```python
from build123d import *

# Parameters (mm, degrees)
F0_R     = 32.397128
F1_DEPTH = 25.4


with BuildPart() as f1:
    # F0 (on Top) → F1 (new body)
    with BuildSketch(Plane.XY):
        with Locations((37.62687, 37.525859)):
            Circle(F0_R)
        with BuildLine():
            ThreePointArc((64.038143, 27.863669), (55.546064, 15.850626), (42.150506, 9.768879))
            Line((42.150506, 9.768879), (57.342436, 32.889675))
            Line((57.342436, 32.889675), (17.938334, 32.889675))
            Line((17.938334, 32.889675), (33.3534, 9.729264))
            ThreePointArc((33.3534, 9.729264), (19.800834, 15.773947), (11.211487, 27.874912))
            ThreePointArc((11.211487, 27.874912), (12.920461, 33.797806), (15.938562, 39.172963))
            Line((15.938562, 39.172963), (18.579211, 37.471808))
            Line((18.579211, 37.471808), (16.513879, 39.937897))
            ThreePointArc((16.513879, 39.937897), (18.978485, 42.682726), (21.79693, 45.062799))
            Line((21.79693, 45.062799), (26.786907, 39.067749))
            Line((26.786907, 39.067749), (23.196478, 46.021628))
            ThreePointArc((23.196478, 46.021628), (25.839836, 47.508267), (28.634337, 48.686485))
            Line((28.634337, 48.686485), (32.258701, 40.739689))
            Line((32.258701, 40.739689), (30.639012, 49.313462))
            ThreePointArc((30.639012, 49.313462), (33.597866, 49.936093), (36.608049, 50.221194))
            Line((36.608049, 50.221194), (37.62687, 40.739689))
            Line((37.62687, 40.739689), (38.795932, 50.214806))
            ThreePointArc((38.795932, 50.214806), (41.991078, 49.881953), (45.123374, 49.168886))
            Line((45.123374, 49.168886), (43.950234, 40.363967))
            Line((43.950234, 40.363967), (47.166887, 48.482341))
            ThreePointArc((47.166887, 48.482341), (50.007564, 47.205017), (52.680711, 45.60649))
            Line((52.680711, 45.60649), (49.80769, 39.289203))
            Line((49.80769, 39.289203), (54.008956, 44.642557))
            ThreePointArc((54.008956, 44.642557), (56.579737, 42.376606), (58.840087, 39.800898))
            Line((58.840087, 39.800898), (56.954861, 37.193418))
            Line((56.954861, 37.193418), (59.273398, 39.222249))
            ThreePointArc((59.273398, 39.222249), (62.317727, 33.820639), (64.038143, 27.863669))
        make_face(mode=Mode.SUBTRACT)
        Polygon((50.473832, 29.364996), (37.623877, 10.928214), (25.100218, 29.364996), align=None, mode=Mode.SUBTRACT)
        with BuildLine():
            ThreePointArc((9.888466, 32.889675), (9.506726, 37.939073), (10.036667, 42.975074))
            Line((10.036667, 42.975074), (14.097949, 40.358721))
            ThreePointArc((14.097949, 40.358721), (11.722598, 36.776711), (9.888466, 32.889675))
        make_face(mode=Mode.SUBTRACT)
        with BuildLine():
            Line((15.116865, 41.605987), (10.986651, 46.537627))
            ThreePointArc((10.986651, 46.537627), (12.544169, 50.244796), (14.614464, 53.691946))
            Line((14.614464, 53.691946), (20.571624, 46.534904))
            ThreePointArc((20.571624, 46.534904), (17.691328, 44.239676), (15.116865, 41.605987))
        make_face(mode=Mode.SUBTRACT)
        with BuildLine():
            Line((22.339414, 47.681575), (17.461614, 57.12881))
            ThreePointArc((17.461614, 57.12881), (20.008646, 59.446429), (22.819841, 61.435378))
            Line((22.819841, 61.435378), (27.907935, 50.279199))
            ThreePointArc((27.907935, 50.279199), (25.056396, 49.124611), (22.339414, 47.681575))
        make_face(mode=Mode.SUBTRACT)
        with BuildLine():
            Line((30.320273, 51.000694), (27.882156, 63.906795))
            ThreePointArc((27.882156, 63.906795), (31.370616, 64.944329), (34.963852, 65.522672))
            Line((34.963852, 65.522672), (36.42892, 51.88823))
            ThreePointArc((36.42892, 51.88823), (33.351504, 51.603405), (30.320273, 51.000694))
        make_face(mode=Mode.SUBTRACT)
        with BuildLine():
            ThreePointArc((64.949322, 44.188954), (65.731013, 38.560434), (65.365273, 32.889675))
            ThreePointArc((65.365273, 32.889675), (63.436107, 36.944067), (60.918471, 40.661766))
            Line((60.918471, 40.661766), (64.949322, 44.188954))
        make_face(mode=Mode.SUBTRACT)
        with BuildLine():
            ThreePointArc((60.860282, 53.372682), (62.672999, 50.316661), (64.08591, 47.056463))
            Line((64.08591, 47.056463), (60.141393, 41.600751))
            ThreePointArc((60.141393, 41.600751), (57.800984, 44.021736), (55.201862, 46.162587))
            Line((55.201862, 46.162587), (60.860282, 53.372682))
        make_face(mode=Mode.SUBTRACT)
        with BuildLine():
            Line((39.00146, 51.880582), (40.679739, 65.482847))
            ThreePointArc((40.679739, 65.482847), (43.933359, 64.932818), (47.100156, 64.005475))
            Line((47.100156, 64.005475), (45.35284, 50.891126))
            ThreePointArc((45.35284, 50.891126), (42.203966, 51.557985), (39.00146, 51.880582))
        make_face(mode=Mode.SUBTRACT)
        with BuildLine():
            ThreePointArc((52.325572, 61.502126), (55.244605, 59.446822), (57.879741, 57.038276))
            Line((57.879741, 57.038276), (53.469349, 47.340571))
            ThreePointArc((53.469349, 47.340571), (50.71484, 48.877102), (47.813072, 50.113221))
            Line((47.813072, 50.113221), (52.325572, 61.502126))
        make_face(mode=Mode.SUBTRACT)
    extrude(amount=F1_DEPTH)


solid = f1.part
```
Check sheet for the modelled part. Datum: model origin and axes. Units: mm. Round coordinates to 2 decimals unless told otherwise and drop trailing zeros. Loops run counter-clockwise (first coordinate to the right, second up) from the corner with the lowest first, then second, coordinate; pieces in that order, holes last. Notation, with made-up numbers: (13, 76) -> (48, 76) arc R36 cw to (48, 114) -> close; hole circle Ø3 at (25, 66.25). An arc over 180 degrees is marked (long way). Answer in a Markdown table with one row per item.
Q1. Release check for a two-part mould opening along Y. For faces 1 (the face through (17.73, 44.274, 12.522)), 2 (the face through (49.64, 21.17, 12.52)), 3 (the face through (37, 31, 0)) record: released by +Y, released by -Y, zero draft, split by the parting line, or undercut.
Data:
| item | result |
|---|---|
| face 1 | undercut |
| face 2 | undercut |
| face 3 | zero draft |
Q2. Sectioned sample at A-A on y = 35.5. Enter the section's corners in (x, z), then the cut area to 3 significant figures.
Data:
| item | result |
|---|---|
| outline | (5.29, 0) -> (9.58, 0) -> (9.58, 25.4) -> (5.29, 25.4) -> close; (11.04, 0) -> (13.7, 0) -> (13.7, 25.4) -> (11.04, 25.4) -> close; (61.54, 0) -> (64.21, 0) -> (64.21, 25.4) -> (61.54, 25.4) -> close; (65.68, 0) -> (69.96, 0) -> (69.96, 25.4) -> (65.68, 25.4) -> close |
| area | 353 mm^2 |
Q3. Sectioned sample at B-B on y = 20. Enter the section's corners in (x, z), then the cut area to 3 significant figures.
Data:
| item | result |
|---|---|
| outline | (10.38, 0) -> (15.63, 0) -> (15.63, 25.4) -> (10.38, 25.4) -> close; (26.52, 0) -> (31.46, 0) -> (31.46, 25.4) -> (26.52, 25.4) -> close; (43.95, 0) -> (48.87, 0) -> (48.87, 25.4) -> (43.95, 25.4) -> close; (59.62, 0) -> (64.87, 0) -> (64.87, 25.4) -> (59.62, 25.4) -> close |
| area | 518 mm^2 |
Q4. Sectioned sample at C-C on z = 10.5. Give the number of separate pieces and of enclosed holes in the cut face, then the cut area to 3 significant figures.
Data:
| item | result |
|---|---|
| separate pieces | 1 |
| enclosed holes | 10 |
| area | 1,580 mm^2 |
Q5. Thickness scan on L1, parallel to X at y = 12, z = 12; L2, parallel to X at y = 40, z = 10.5; L3, parallel to Y at x = 21.5, z = 10. Record the ranges inside material, lowest first.
Data:
| item | result |
|---|---|
| L1 | x = 17.68 to 25.82, 31.84 to 36.9, 38.37 to 43.62, 49.43 to 57.58 |
| L2 | x = 5.32 to 9.61, 13.83 to 16.56, 26.01 to 26.31, 50.13 to 50.37, 58.69 to 61.43, 65.64 to 69.93 |
| L3 | y = 9.43 to 14.49, 27.54 to 32.89, 44.84 to 49.31, 60.57 to 65.62 |
Q6. Go/stop test with flat-tipped pins: P1, Ø8, axis at y = 57, z = 16.5, coming from the -X side; P2, Ø12.5, axis at x = 44.5, z = 13, coming from the +Y side; P3, Ø12, axis at y = 27.5, z = 4.5, coming from the +X side. Record where each tip stops, or that it passes through.
Data:
| item | result |
|---|---|
| P1 | stops at x = 9.16 |
| P2 | stops at y = 69.92 |
| P3 | stops at x = 69.77 |
